```python
from build123d import *

# Parameters (mm, degrees)
SKETCH1_R           = 37.5
BOSS_EXTRUDE1_DEPTH = 100
SKETCH2_R           = 31.5
CUT_EXTRUDE1_DEPTH  = 6.5
SKETCH3_R           = 52.959705575
BOSS_EXTRUDE2_DEPTH = 90


with BuildPart() as part:
    # Sketch1 → Boss-Extrude1 (new body)
    with BuildSketch(Plane.XY):
        Circle(SKETCH1_R)
    extrude(amount=BOSS_EXTRUDE1_DEPTH)

    # Sketch2 → Cut-Extrude1 (cut)
    with BuildSketch(Plane.XY.offset(100)):
        Circle(SKETCH2_R)
    extrude(amount=-CUT_EXTRUDE1_DEPTH, mode=Mode.SUBTRACT)

    # Sketch3 → Boss-Extrude2 (add)
    with BuildSketch(Plane(origin=(0, 0, 0), x_dir=(-1, 0, 0), z_dir=(0, 0, -1))):
        Circle(SKETCH3_R)
    extrude(amount=-BOSS_EXTRUDE2_DEPTH)


solid = part.part
```
Geometry check sheet. Reference: the model listing, model coordinates, mm. A direction names the side the tool comes from. Coordinates: 2 decimals unless noted, no trailing zeros. Write each loop counter-clockwise with the first axis right and the second up, starting at its lowest first coordinate (ties: lowest second). Pieces come first, ordered by that corner, then holes. Notation, with made-up numbers: M 38.25,57 L 86.25,57 A13 ccw 86.25,82 Z; hole C 79.5,-15 d2. An arc over 180 degrees is marked long. Answer as a JSON object with one key per item and string values.
1. Section check A-A, the plane x = 0. Enter the section's corners in (y, z), plus the area to 3 significant figures.
Answers below:
{"outline": "M -52.96,0 L 52.96,0 L 52.96,90 L 37.5,90 L 37.5,100 L 31.5,100 L 31.5,93.5 L -31.5,93.5 L -31.5,100 L -37.5,100 L -37.5,90 L -52.96,90 Z", "area": "9,870 mm²"}
2. Draft check along Y on faces 3 (the flat face through (-9, 31, 100)), 4 (the cylindrical face through (-4.88, 37.18, 94.93)), 5 (the cylindrical face through (-4.101, 31.232, 96.796)). Enter one of: released by +Y, released by -Y, zero draft, split by the parting line, or undercut.
Answers below:
{"face 3": "zero draft", "face 4": "split by the parting line", "face 5": "undercut"}
3. Tool access check on faces 1 (the flat face through (36.05, -11.03, 90)), 2 (the flat face through (1, 1, 0)). Record the directions out of +Z, -Z, +X, -X, +Y, -Y that give a thin tool (end or side, any length) a straight path to the whole face; none if there is none.
Answers below:
{"face 1": "+Z", "face 2": "-Z, +X, -X, +Y, -Y"}
4. Scan lines: L1, parallel to Y at x = 0, z = 98; L2, parallel to Z at x = -42, y = 10; L3, parallel to Z at x = -27, y = -4. Record each from-to range of solid material in increasing order.
Answers below:
{"L1": "y = -37.5 to -31.5, 31.5 to 37.5", "L2": "z = 0 to 90", "L3": "z = 0 to 93.5"}
5. Section check D-D, the plane x = -33.5. Enter the section's corners in (y, z).
Answers below:
{"outline": "M -41.02,0 L 41.02,0 L 41.02,90 L 16.85,90 L 16.85,100 L -16.85,100 L -16.85,90 L -41.02,90 Z"}
6. Go/stop test with flat-tipped pins: pin 1 Ø6 at (y, z) = (-26, 27.5) entering from -X; pin 2 Ø10 at (x, y) = (-17.5, 6) entering from +Z; pin 3 Ø1.5 at (y, z) = (11.5, 55) entering from -X. Record where each tip stops, or that it passes through.
Answers below:
{"pin 1": "stops at x = -47.7", "pin 2": "stops at z = 93.5", "pin 3": "stops at x = -51.86"}
7. Section check C-C, the plane z = 85.5. Enter the section's corners in (x, y).
Answers below:
{"outline": "C 0,0 d105.92"}
